Autodesk Inventor part; units mm, degrees
ref_plane "YZ Plane" through (0, 0, 0) normal (1, 0, 0) x (0, 1, 0)
ref_plane "XZ Plane" through (0, 0, 0) normal (0, 1, 0) x (-1, 0, 0)
ref_plane "XY Plane" through (0, 0, 0) normal (0, 0, 1) x (1, 0, 0)
sketch "Sketch1" plane through (0, 0, 0) normal (0, 1, 0) x (-1, 0, 0)
  circle A0 centre (0, 0) radius 6.5
  line L0 (7.3246, 1.5) -> (6.3246, 1.5)
  line L1 (6.3246, 1.5) -> (6.3246, -1.5)
  line L2 (6.3246, -1.5) -> (7.3246, -1.5)
  line L3 (7.3246, -1.5) -> (7.3246, 1.5)
  dimension "d0" = 13
  dimension "d8" = 1
  dimension "d9" = 3
extrude "Extrusion1" add sketch "Sketch1" along normal blind 17
sketch "Sketch2" plane through (0, 0, 0) normal (0, -1, 0) x (0, 0, -1)
  circle A0 centre (0, 0) radius 10
  dimension "d3" = 20
extrude "Extrusion2" add sketch "Sketch2" along normal blind 1.5
sketch "Sketch4" plane through (0, 17, 0) normal (0, 1, 0) x (1, 0, 0)
  circle A0 centre (0, 0) radius 6
  dimension "d10" = 12
extrude "Extrusion3" add sketch "Sketch4" along normal blind 10
sketch "Sketch5" plane through (0, 27, 0) normal (0, 1, 0) x (1, 0, 0)
  point P0 (0, 0)
  point P1 (0, 0)
hole "Hole1" at (0, 27, 0) direction (0, -1, 0) diameter 3.8 depth 10 tip angle 118
sketch "Sketch6" plane through (0, 0, 0) normal (0, 0, 1) x (1, 0, 0)
  circle A0 centre (0, 23) radius 0.75
  line L0 (6, 27) -> (-6, 27)
  line L1 (0, -7.2) -> (0, 32.7)
  point P0 (0, 0)
  dimension "d21" = 1.5
  dimension "d26" = 4
extrude "Extrusion4" cut sketch "Sketch6" against normal up to surface
properties part number "wheel_adapt"
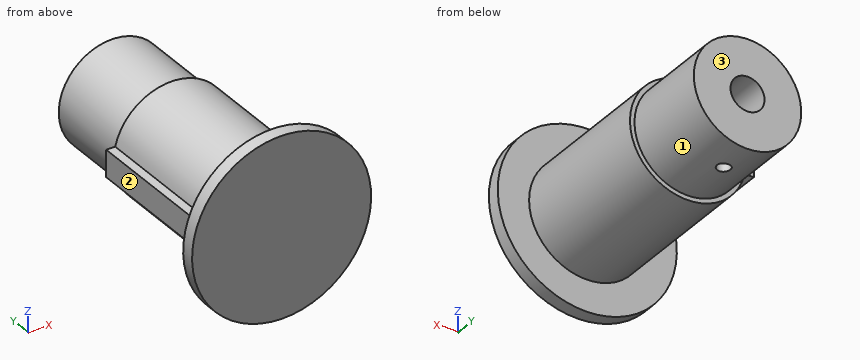
Can you work these out from the model? Positions are in its coordinate system, mm. Face numbers are marked on the shaded views. A direction names the side the tool comes from. Coordinates: 2 decimals unless noted, no trailing zeros. Write each loop counter-clockwise with the first axis right and the second up, starting at its lowest first coordinate (ties: lowest second). Pieces come first, ordered by that corner, then holes. Notation, with made-up numbers: M 57.5,76 L 111.5,76 A12 ccw 111.5,95 Z; hole C 54,-33.5 d5. An arc over 180 degrees is marked long. Use one line per item in the form item = value.
Q1. I need wall thicknesses on line 1 along X through (y, z) = (23, 0); line 2 along Y through (x, z) = (0, -4.6). Which ranges of each line are inside material? Lowest first, please. Write a range as from..to.
Model answer:
line_1 = -6..-1.9, 1.9..6
line_2 = -1.5..22.25, 23.75..27
Q2. For the marked faces 1, 2 and 3, which set-ups out of +Z, -Z, +X, -X, +Y, -Y let a thin tool reach every point of the face, with its end or its side?
Model answer:
face_1 = +Y
face_2 = +Z, -Z, -X, +Y
face_3 = +Z, -Z, +X, -X, +Y
Q3. If we section it at D-D (y = 9.5): Write out the boundary of the cut face in (x, z).
Model answer:
outline = M -7.32,-1.5 L -6.32,-1.5 A6.5 ccw long -6.32,1.5 L -7.32,1.5 Z
Q4. For P1, Ø3.5, axis at y = 9, z = -0.5, coming from the -X side; P2, Ø12, axis at x = -3.5, y = 5.5, coming from the +Z side; P3, Ø10, axis at y = 17.5, z = -5, coming from the +X side; P4, Ø1, axis at y = 18, z = -7, coming from the +X side, each with a flat end and sliding along its axis, tell me the tip position at first contact or that it passes through.
Model answer:
P1 = -7.32
P2 = 9.94
P3 = 6.5
P4 = through
Q5. If we section it at B-B (y = 24.5): Write out the boundary of the cut face in (x, z), then the cut area to 3 significant figures.
Model answer:
outline = C 0,0 d12; hole C 0,0 d3.8
area = 102 mm^2
Q6. If we section it at A-A (x = -5.25): Write out the boundary of the cut face in (y, z), then the cut area to 3 significant figures.
Model answer:
outline = M -1.5,-8.51 L 0,-8.51 L 0,-3.83 L 17,-3.83 L 17,-2.9 L 27,-2.9 L 27,2.9 L 17,2.9 L 17,3.83 L 0,3.83 L 0,8.51 L -1.5,8.51 Z
area = 214 mm^2
Q7. If we section it at C-C (z = 4.5): Write out the boundary of the cut face in (x, y), then the cut area to 3 significant figures.
Model answer:
outline = M -8.93,-1.5 L 8.93,-1.5 L 8.93,0 L 4.69,0 L 4.69,17 L 3.97,17 L 3.97,27 L -3.97,27 L -3.97,17 L -4.69,17 L -4.69,0 L -8.93,0 Z
area = 266 mm^2
